CAD build for the part. Positions are in the model's coordinates, mm. A direction names the side the tool comes from. Round coordinates to 2 decimals unless told otherwise and drop trailing zeros. Order: outer loops, then holes, each group sorted by start corner. A loop starts at its lowest first (then second) coordinate and runs counter-clockwise, first axis right, second up. Notation, with made-up numbers: (-4.5, -35.5) -> (6.5, -35.5) arc R18 cw to (6.5, -26.5) -> close; hole circle Ø6 at (-14, -34.5). An arc over 180 degrees is marked (long way). Return JSON: item names as keys, results as strings. Group by question number.
Q1. Cut at A-A (y = 0). Write the cut outline in (x, z), then the cut area to 3 significant figures.
Q2. Cut at C-C (z = 0). Write the cut outline in (x, y).
Q3. Cut at B-B (x = -1). Write the cut outline in (y, z).
Q4. Which spindle directions (+Z, -Z, +X, -X, +Y, -Y) get a long thin tool onto all of the face, cutting with end or side? Do faces 1 (the flat face through (-4.75, 2, 4.3)), 2 (the cylindrical face through (29.837, -2.681, -6.466)), 3 (the cylindrical face through (-2.34, -2.79, -3.64)). Say none if no direction does.
Q5. Flat gauge pins, fed straight in: pin 1 (1.5 mm diameter, centred on y = 10, z = 3, fed in from +X); pin 2 (12 mm diameter, centred on x = 23.5, y = 10, fed in from -Z); pin 3 (1.1 mm diameter, centred on y = 0, z = -0.5, fed in from +X); pin 4 (2 mm diameter, centred on x = 27, z = -9.5, fed in from +Y). Where does each tip first touch, or does it go through?
Q6. Cut at D-D (x = 28.5). Write the cut outline in (y, z) (3 decimals), then the cut area to 3 significant figures.
Q7. Mould opens along Y. For faces 4 (the flat face through (24.907, -3.1, -6.5)), 5 (the cylindrical face through (12.28, 4.53, -14.38)), 6 (the flat face through (0, 0, 0)) say: +Y half, -Y half, draft (parallel to the pull), parting line (faces both ways), or undercut.
Q8. Probe line 1 along Y through (x, z) = (-1.25, 0); line 2 along X through (y, z) = (-0.5, 12); line 3 along Y through (x, z) = (18, 0). List the from-to ranges inside material, lowest first.
from build123d import *
from build123d.topology import SkipClean

# Parameters (mm, degrees)
SKETCH1_R           = 15.07617
BOSS_EXTRUDE1_DEPTH = 34.9071592
SKETCH2_R           = 9.3853
SKETCH2_R_2         = 4.5847
BOSS_EXTRUDE2_DEPTH = 4.7498
CUT_EXTRUDE1_DEPTH  = 26
SKETCH4_R           = 2.3
CUT_EXTRUDE2_DEPTH  = 2.6
CUT_EXTRUDE3_START  = -10
SKETCH5_R           = 15.07617
SKETCH5_R_2         = 7
CUT_EXTRUDE3_DEPTH  = 10


with BuildPart() as part:
    # Sketch1 → Boss-Extrude1 (new body)
    with BuildSketch(Plane(origin=(0, 0, 0), x_dir=(0, 0, -1), z_dir=(1, 0, 0))):
        Circle(SKETCH1_R)
    extrude(amount=BOSS_EXTRUDE1_DEPTH)

    # Sketch2 → Boss-Extrude2 (add)
    with BuildSketch(Plane.ZY):
        with Locations(Location((0, 0, 0), (0, 0, 180))):
            Circle(SKETCH2_R)
        Circle(SKETCH2_R_2, mode=Mode.SUBTRACT)
    extrude(amount=BOSS_EXTRUDE2_DEPTH)

    # Sketch3 → Cut-Extrude1 (cut)
    with BuildSketch(Plane(origin=(34.9071592, 0, 0), x_dir=(0, 0, -1), z_dir=(1, 0, 0))):
        with BuildLine():
            Line((-1.775, 1.462660248), (1.775, 1.462660248))
            ThreePointArc((1.775, 1.462660248), (0, -2.3), (-1.775, 1.462660248))
        make_face()
    extrude(amount=-CUT_EXTRUDE1_DEPTH, mode=Mode.SUBTRACT)

    # Sketch4 → Cut-Extrude2 (cut)
    with SkipClean():  # the faces are left unmerged after this step: merging them gives an invalid solid
        with BuildSketch(Plane(origin=(34.9071592, 0, 0), x_dir=(0, 0, -1), z_dir=(1, 0, 0))):
            Circle(SKETCH4_R)
        extrude(amount=-CUT_EXTRUDE2_DEPTH, mode=Mode.SUBTRACT)

    # Sketch5 → Cut-Extrude3 (cut)
    with SkipClean():  # the faces are left unmerged after this step: merging them gives an invalid solid
        with BuildSketch(Plane(origin=(34.9071592, 0, 0), x_dir=(0, 0, -1), z_dir=(1, 0, 0)).offset(CUT_EXTRUDE3_START)):
            Circle(SKETCH5_R)
            Circle(SKETCH5_R_2, mode=Mode.SUBTRACT)
        extrude(amount=CUT_EXTRUDE3_DEPTH, mode=Mode.SUBTRACT)


solid = part.part
Solution:
{
 "1": {"outline": "(-4.75, -9.39) -> (0, -9.39) -> (0, -15.08) -> (24.91, -15.08) -> (24.91, -7) -> (34.91, -7) -> (34.91, -2.3) -> (8.91, -2.3) -> (8.91, 2.3) -> (34.91, 2.3) -> (34.91, 7) -> (24.91, 7) -> (24.91, 15.08) -> (0, 15.08) -> (0, 9.39) -> (-4.75, 9.39) -> (-4.75, 4.58) -> (0, 4.58) -> (0, -4.58) -> (-4.75, -4.58) -> close", "area": "817 mm²"},
 "2": {"outline": "(-4.75, -9.39) -> (0, -9.39) -> (0, -15.08) -> (24.91, -15.08) -> (24.91, -7) -> (34.91, -7) -> (34.91, -2.3) -> (8.91, -2.3) -> (8.91, 1.46) -> (32.31, 1.46) -> (32.31, 2.3) -> (34.91, 2.3) -> (34.91, 7) -> (24.91, 7) -> (24.91, 15.08) -> (0, 15.08) -> (0, 9.39) -> (-4.75, 9.39) -> (-4.75, 4.58) -> (0, 4.58) -> (0, -4.58) -> (-4.75, -4.58) -> close"},
 "3": {"outline": "circle Ø18.77 at (0, 0); hole circle Ø9.17 at (0, 0)"},
 "4": {"face 1": "+Z, -Z, -X, +Y, -Y", "face 2": "+X", "face 3": "-X"},
 "5": {"pin 1": "stops at x = 24.91", "pin 2": "stops at z = -14.54", "pin 3": "stops at x = 8.91", "pin 4": "passes through"},
 "6": {"outline": "circle Ø14 at (0, 0); hole (1.463, -1.775) -> (1.463, 1.775) arc R2.3 ccw (long way) to start", "area": "139 mm²"},
 "7": {"face 4": "draft", "face 5": "parting line", "face 6": "undercut"},
 "8": {"line 1": "y = -9.39 to -4.58, 4.58 to 9.39", "line 2": "x = 0 to 24.91", "line 3": "y = -15.08 to -2.3, 1.46 to 15.08"}
}
